```python
from build123d import *

# Parameters (mm, degrees)
ESQUISSE1_R        = 1.75
BOSS_EXTRU_1_DEPTH = 3
CONG_1_R           = 3.5


with BuildPart() as part:
    # Esquisse1 → Boss.-Extru.1 (new body)
    with BuildSketch(Plane.XY):
        Polygon((-10.55794702, -7.3), (-10.19205298, 14.8), (10.19205298, 14.8), (10.55794702, -7.3), align=None)
        with Locations((-6.75, 11.3)):
            Circle(ESQUISSE1_R, mode=Mode.SUBTRACT)
        with Locations((6.75, 11.3)):
            Circle(ESQUISSE1_R, mode=Mode.SUBTRACT)
        with Locations((-7, -3.8)):
            Circle(ESQUISSE1_R, mode=Mode.SUBTRACT)
        with Locations((7, -3.8)):
            Circle(ESQUISSE1_R, mode=Mode.SUBTRACT)
    extrude(amount=BOSS_EXTRU_1_DEPTH)

    # Congé1
    cong_1_edges = [part.edges().sort_by_distance(p)[0] for p in [
        (-10.55794702, -7.3, 1.5),
        (-10.19205298, 14.8, 1.5),
        (10.19205298, 14.8, 1.5),
        (10.55794702, -7.3, 1.5),
    ]]
    fillet(cong_1_edges, radius=CONG_1_R)


solid = part.part
```
CAD build for the part. Positions are in the model's coordinates, mm. Give positions to 0.01 mm unless a question says otherwise; leave off trailing zeros. Write each loop counter-clockwise with the first axis right and the second up, starting at its lowest first coordinate (ties: lowest second). Pieces come first, ordered by that corner, then holes. Notation, with made-up numbers: (-33.5, 26) -> (21.5, 26) arc R15 ccw to (21.5, 35) -> close; hole circle Ø5 at (55.5, -19). An arc over 180 degrees is marked (long way). Write each question's results on one line, items separated by ' | '.
1. Wall check: probe 1 along X at (y, z) = (-3.5, 2.2); probe 2 along Y at (x, z) = (6.75, 1.1); probe 3 along X at (y, z) = (10.5, 0.6). Give the ranges that are in metal, low to high. Write a range as [from, to].
Geometry check:
probe 1: [-10.5, -8.72], [-5.28, 5.28], [8.72, 10.5] | probe 2: [-7.3, -5.53], [-2.07, 9.55], [13.05, 14.8] | probe 3: [-10.26, -8.31], [-5.19, 5.19], [8.31, 10.26]
2. Cut at C-C, the plane x = -5.5. Write the cut outline in (y, z), then the cut area to 3 significant figures.
Geometry check:
outline: (-7.3, 0) -> (-4.7, 0) -> (-4.7, 3) -> (-7.3, 3) -> close; (-2.9, 0) -> (10.08, 0) -> (10.08, 3) -> (-2.9, 3) -> close; (12.52, 0) -> (14.8, 0) -> (14.8, 3) -> (12.52, 3) -> close | area: 53.5 mm²
3. Drop flat-ended pins along their axis: P1, Ø2, axis at x = 7, y = -3.8, coming from the -Z side; P2, Ø1.5, axis at y = 9, z = 0.5, coming from the +X side. Give the stop position or say it passes through.
Geometry check:
P1: through | P2: x = 10.3
4. Cut at A-A, the plane z = 2.4. Write the cut outline in (x, y).
Geometry check:
outline: (-10.5, -3.74) arc R3.5 ccw to (-7, -7.3) -> (7, -7.3) arc R3.5 ccw to (10.5, -3.74) -> (10.25, 11.36) arc R3.5 ccw to (6.75, 14.8) -> (-6.75, 14.8) arc R3.5 ccw to (-10.25, 11.36) -> close; hole circle Ø3.5 at (-7, -3.8); hole circle Ø3.5 at (-6.75, 11.3); hole circle Ø3.5 at (6.75, 11.3); hole circle Ø3.5 at (7, -3.8)
5. Cut at D-D, the plane y = -6. Write the cut outline in (x, z), then the cut area to 3 significant figures.
Geometry check:
outline: (-9.72, 0) -> (9.72, 0) -> (9.72, 3) -> (-9.72, 3) -> close | area: 58.3 mm²
6. Cut at B-B, the plane y = 10.75. Write the cut outline in (x, z), then the cut area to 3 significant figures.
Geometry check:
outline: (-10.26, 0) -> (-8.41, 0) -> (-8.41, 3) -> (-10.26, 3) -> close; (-5.09, 0) -> (5.09, 0) -> (5.09, 3) -> (-5.09, 3) -> close; (8.41, 0) -> (10.26, 0) -> (10.26, 3) -> (8.41, 3) -> close | area: 41.6 mm²
7. Two-plate mould, pull along X, no slides. Class faces 1 (the flat face through (0, -7.3, 1)), 2 (the cylindrical face through (9.47, -6.28, 1.52)), 3 (the cylindrical face through (-6.978, 13.035, 1.479)): pulls with the +X half, pulls with the -X half, needs draft (parallel to the pull), parting line crosses it, or undercut.
Geometry check:
face 1: needs draft | face 2: pulls with the +X half | face 3: undercut
